Verification items for the finished model (mm, model axes). A direction names the side the tool comes from. Coordinates: 2 decimals unless noted, no trailing zeros. Order: outer loops, then holes, each group sorted by start corner. A loop starts at its lowest first (then second) coordinate and runs counter-clockwise, first axis right, second up. Notation, with made-up numbers: M 10,-6 L 64,-6 A5 cw 64,0 Z; hole C -31,71.25 d1. An arc over 180 degrees is marked long. Return JSON: item names as keys, results as strings. Group by question number.
1. Section check B-B, the plane z = 137. Give the number of separate pieces and of enclosed holes in the cut face, plus the area to 3 significant figures.
2. Set-up check for faces 5 (the flat face through (28.01, -9.46, 125.44)), 6 (the flat face through (19, -41, 0)), 7 (the flat face through (19, -68, 25.4)): record each of +Z, -Z, +X, -X, +Y, -Y from which the full face is reachable in a straight line by a thin tool's end or side.
3. Material ranges on line 1 along Y through (x, z) = (19.05, 6.25); line 2 along Y through (x, z) = (21, 21.5); line 3 along X through (y, z) = (-12.5, 13.5), recorded low to high.
4. Section check A-A, the plane y = -22. Record the cut outline in (x, z), plus the area to 3 significant figures.
5. Mould release check, pull along Y, two halves, no side actions. Record for faces 1 (the flat face through (29, -41, 153.365)), 2 (the flat face through (19, -82.55, 78)), 3 (the cylindrical face through (17.68, -77.057, 133.321)), 4 (the flat face through (19, 0, 78)): +Y half, -Y half, draft (parallel to the pull), parting line (faces both ways), or undercut.
6. Gauge pin test, flat ends, axial feed: pin 1 (2 mm diameter, centred on y = -52, z = 59, fed in from -X); pin 2 (1.5 mm diameter, centred on x = 5.5, y = -63, fed in from +Z). Record the tip position at first contact, or that the pin passes through.
```python
from build123d import *

# Parameters (mm, degrees)
F1_DEPTH = 82.55
F2_R     = 4.36499
F3_DEPTH = 25.4
F4_R     = 4.3688
F5_DEPTH = 25.4


with BuildPart() as f1:
    # F0 (on Front) → F1 (new body)
    with BuildSketch(Plane.XZ):
        Polygon((0, 133.35), (0, 0), (38.1, 0), (38.1, 153.3652), (20.0152, 153.3652), align=None)
    extrude(amount=F1_DEPTH)

    # F2 (on face) → F3 (cut)
    with BuildSketch(Plane(origin=(-66.675, 0, 66.675), x_dir=(0, -1, 0), z_dir=(-0.707107, 0, 0.707107))):
        with Locations((9.525, 108.445573)):
            Circle(F2_R)
        with Locations((73.025, 108.445573)):
            Circle(F2_R)
    extrude(amount=-F3_DEPTH, mode=Mode.SUBTRACT)

    # F4 (on face) → F5 (cut)
    with BuildSketch(Plane(origin=(0, 0, 0), x_dir=(1, 0, 0), z_dir=(0, 0, -1))):
        with BuildLine():
            ThreePointArc((23.4188, 14.15288), (15.960792, 17.242088), (19.05, 9.78408))
            ThreePointArc((19.05, 9.78408), (22.139208, 11.063672), (23.4188, 14.15288))
        make_face()
        with Locations((19.05, 68.39712)):
            Circle(F4_R)
    extrude(amount=-F5_DEPTH, mode=Mode.SUBTRACT)


solid = f1.part
```
Answers follow:
{
 "1": {"separate pieces": "1", "enclosed holes": "2", "area": "2,670 mm^2"},
 "2": {"face 5": "none", "face 6": "-Z, +X, -X, +Y, -Y", "face 7": "-Z"},
 "3": {"line 1": "-82.55 to -72.77, -64.03 to -18.52, -9.78 to 0", "line 2": "-82.55 to -72.31, -64.49 to -18.06, -10.24 to 0", "line 3": "0 to 15.01, 23.09 to 38.1"},
 "4": {"outline": "M 0,0 L 38.1,0 L 38.1,153.37 L 20.02,153.37 L 0,133.35 Z", "area": "5,640 mm^2"},
 "5": {"face 1": "draft", "face 2": "-Y half", "face 3": "undercut", "face 4": "+Y half"},
 "6": {"pin 1": "x = 0", "pin 2": "z = 139.6"}
}
